from build123d import *


with BuildPart() as f1:
    # F0 (on Top) → F1 (revolve)
    with BuildSketch(Plane.XY):
        with BuildLine():
            Line((22, -10), (12.35, 0))
            Line((12.35, 0), (10.35, 0))
            Line((10.35, 0), (20.422777, -9.458007))
            ThreePointArc((20.422777, -9.458007), (21.055595, -9.859572), (21.791797, -10))
            Line((21.791797, -10), (22, -10))
        make_face()
        Polygon((2.037337, 0), (10.35, 0), (10.35, 1), (1.35, 1), (1.35, 0), align=None)
        Polygon((10.35, 0), (12.35, 0), (12.35, 3), (10.35, 3), (10.35, 1), align=None)
        Polygon((10.35, 3), (12.35, 3), (11.049551, 3.974945), (10.35, 4), align=None)
    revolve(axis=Axis((0, -5, 0), (0, -1, 0)))


solid = f1.part
CAD build for the part. Positions are in the model's coordinates, mm. A direction names the side the tool comes from. Round coordinates to 2 decimals unless told otherwise and drop trailing zeros. Write each loop counter-clockwise with the first axis right and the second up, starting at its lowest first coordinate (ties: lowest second). Pieces come first, ordered by that corner, then holes.
(1) Drop flat-ended pins along their axis: P1, Ø3, axis at x = -9, y = -4, coming from the -Z side; P2, Ø1, axis at y = -7.5, z = 0, coming from the -X side; P3, Ø4.5, axis at x = 0, z = 0, coming from the -Y side; P4, Ø10, axis at x = 10, z = -11.5, coming from the +Y side. Give the stop position or say it passes through.
(2) Slice it at B-B, the plane z = 0. Write the cut outline in (x, y).
(3) 3-axis set-ups, long thin cutter, end or side, ignore diameter. For faces 3 (the face through (0, 1, -2)), 4 (the face through (-0.29, 0.49, -1.32)), 5 (the face through (0, 0, -2)): which of +Z, -Z, +X, -X, +Y, -Y reach the whole face in a straight line?
(4) Probe line 1 along Z through (x, y) = (0, 2.8); line 2 along Z through (x, y) = (0, 0.7); line 3 along Y through (x, z) = (1.5, 9). List the from-to ranges inside material, lowest first.
(5) Slice it at C-C, the plane y = -5. Write the cut outline in (x, z) (3 decimals).
(6) Mould opens along X. For faces 1 (the face through (-2.38, -0.59, -10.72)), 2 (the face through (11.78, 1.52, 3.71)) say: pulls with the +X half, pulls with the -X half, needs draft (parallel to the pull), parting line crosses it, or undercut.
(7) Slice it at A-A, the plane x = 0. Write the cut outline in (y, z), and give its area (3 significant figures).
From the geometry:
1. P1: stops at z = -15.4
1. P2: stops at x = -20.07
1. P3: stops at y = 0
1. P4: stops at y = 4
2. outline: (-22, -10) - (-21.79, -10) arc R2 ccw to (-20.42, -9.46) - (-10.35, 0) - (-1.35, 0) - (-1.35, 1) - (-10.35, 1) - (-10.35, 4) - (-11.05, 3.97) - (-12.35, 3) - (-12.35, 0) - close; (1.35, 0) - (10.35, 0) - (20.42, -9.46) arc R2 ccw to (21.79, -10) - (22, -10) - (12.35, 0) - (12.35, 3) - (11.05, 3.97) - (10.35, 4) - (10.35, 1) - (1.35, 1) - close
3. face 3: +Y
3. face 4: +Y, -Y
3. face 5: -Y
4. line 1: z = -12.35 to -10.35, 10.35 to 12.35
4. line 2: z = -12.35 to -1.35, 1.35 to 12.35
4. line 3: y = 0 to 1
5. outline: circle Ø34.35 at (0, 0); hole circle Ø31.35 at (0, 0)
6. face 1: undercut
6. face 2: parting line crosses it
7. outline: (-10, -22) - (0, -12.35) - (3, -12.35) - (3.97, -11.05) - (4, -10.35) - (1, -10.35) - (1, -1.35) - (0, -1.35) - (0, -10.35) - (-9.46, -20.42) arc R2 ccw to (-10, -21.79) - close; (-10, 21.79) arc R2 ccw to (-9.46, 20.42) - (0, 10.35) - (0, 1.35) - (1, 1.35) - (1, 10.35) - (4, 10.35) - (3.97, 11.05) - (3, 12.35) - (0, 12.35) - (-10, 22) - close
7. area: 62.5 mm2
